Source: CAD feature listing. Evaluate the final solid. Frame: model axes, mm. A direction names the side the tool comes from. Coordinates: 2 decimals unless noted, no trailing zeros. Loops run counter-clockwise (first coordinate to the right, second up) from the corner with the lowest first, then second, coordinate; pieces in that order, holes last. Notation, with made-up numbers: M -27,0.5 L 27,0.5 A22 cw 27,19.5 Z; hole C -9,-26.5 d9. An arc over 180 degrees is marked long. One line per question, with ' | ' between items. Start each with the question number.
1. Pin query (flat end, axial travel): P1, Ø3, axis at x = 0, y = 0, coming from the +Z side; P2, Ø3, axis at y = -1.5, z = -113.5, coming from the -X side; P3, Ø1, axis at x = -2, y = 0.5, coming from the -Z side; P4, Ø1.7, axis at y = -0.5, z = -125, coming from the -X side. Return the tip coordinate at first contact, or that it passes through.
2. Section query B-B, the plane x = 0. Output: boundary loops of the cut face in (y, z).
3. Ray query, probe 1 along Y at (x, z) = (-0.3, -125); probe 2 along X at (y, z) = (0.2, -20.5); probe 3 along Y at (x, z) = (0, -22). Return the intervals inside material, ascending.
4. Section query A-A, the plane y = 0. Output: boundary loops of the cut face in (x, z), and give its area (3 significant figures).
5. Mould query, pull axis Y, two halves, no side actions, for faces 1 (the cylindrical face through (-3, 0, -63)), 2 (the flat face through (0, 0, -128)), 3 (the cylindrical face through (-0.54, -2.44, -54.23)). Classes: pulls with the +Y half, pulls with the -Y half, needs draft (parallel to the pull), parting line crosses it, or undercut.
6. Access query for faces 4 (the flat face through (0, 0, -110)), 5 (the flat face through (2, 0, -122)), 6 (the cylindrical face through (0, 0, -126)), 7 (the flat face through (-2, 2, 0)), 8 (the flat face through (-1, -1.3, -125)). Directions: +Z, -Z, +X, -X, +Y, -Y. A direction counts if a zero-diameter tool reaches every point of the face in a straight line with its end or side. Return the directions, or none.
7. Section query C-C, the plane z = -95. Output: boundary loops of the cut face in (x, y).
```python
from build123d import *

# Parameters (mm, degrees)
F0_R     = 3
F1_DEPTH = 128
F2_R     = 2.5
F3_DEPTH = 110
F4_W     = 3.289427
F4_H     = 6.793895
F4_W_2   = 3.708657
F4_H_2   = 6.848642
F5_DEPTH = 12.5
F6_R     = 1
F7_DEPTH = 25


with BuildPart() as f1:
    # F0 (on Top) → F1 (new body)
    with BuildSketch(Plane.XY):
        Circle(F0_R)
    extrude(amount=-F1_DEPTH)

    # F2 (on face) → F3 (cut)
    with BuildSketch(Plane.XY):
        Circle(F2_R)
    extrude(amount=-F3_DEPTH, mode=Mode.SUBTRACT)

    # F4 (on Front) → F5 (cut, symmetric)
    with BuildSketch(Plane.XZ):
        with Locations((2.644713, -125.396947)):
            Rectangle(F4_W, F4_H)
        with Locations((-2.854328, -125.424321)):
            Rectangle(F4_W_2, F4_H_2)
    extrude(amount=F5_DEPTH, both=True, mode=Mode.SUBTRACT)

    # F6 (on face) → F7 (cut)
    with BuildSketch(Plane(origin=(-1, 0, 0), x_dir=(0, -1, 0), z_dir=(-1, 0, 0))):
        with Locations((0, -125)):
            Circle(F6_R)
    extrude(amount=-F7_DEPTH, mode=Mode.SUBTRACT)


solid = f1.part
```
Taken from the geometry:
1) P1: z = -110 | P2: x = -3 | P3: z = -122 | P4: x = -1
2) outline: M -3,-128 L 3,-128 L 3,0 L 2.5,0 L 2.5,-110 L -2.5,-110 L -2.5,0 L -3,0 Z; hole C 0,-125 d2
3) probe 1: -2.98 to -1, 1 to 2.98 | probe 2: -2.99 to -2.49, 2.49 to 2.99 | probe 3: -3 to -2.5, 2.5 to 3
4) outline: M -3,-122 L -1,-122 L -1,-124 L 1,-124 L 1,-122 L 3,-122 L 3,0 L 2.5,0 L 2.5,-110 L -2.5,-110 L -2.5,0 L -3,0 Z; M -1,-128 L 1,-128 L 1,-126 L -1,-126 Z | area: 190 mm^2
5) face 1: parting line crosses it | face 2: needs draft | face 3: undercut
6) face 4: +Z | face 5: -Z, +X, +Y, -Y | face 6: +X, -X | face 7: +Z, +X, -X, +Y, -Y | face 8: -Z, -X, +Y, -Y
7) outline: C 0,0 d6; hole C 0,0 d5
